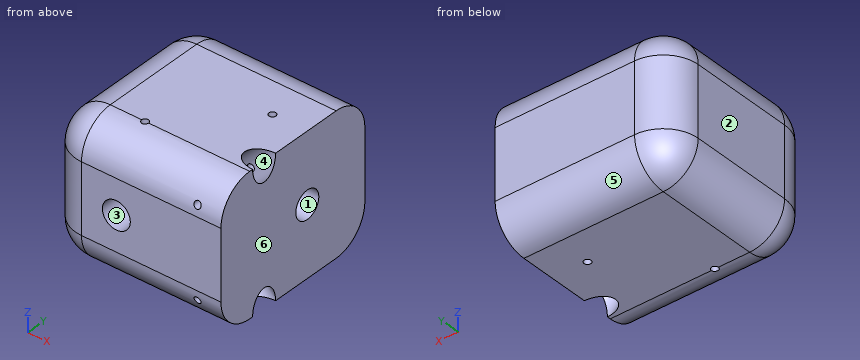
from build123d import *

# Parameters (mm, degrees)
F0_W          = 30
F0_H          = 30
F1_DEPTH      = 20
F2_R          = 2
F3_DEPTH      = 15
F4_R          = 2
F4_R_2        = 0.5
F5_DEPTH      = 15
F7_R          = 2
F8_DEPTH      = 15
F10_R         = 2
F11_DEPTH     = 15
F12_R         = 0.5
F13_DEPTH     = 20.0010001
F14_T1_DEPTH  = 10
F14_T3_DEPTH  = 32.5
F14_T5_DEPTH  = 15
F14_S9_W      = 5
F14_S9_H      = 5
F14_T10_DEPTH = 5
F14_S15_W     = 5
F14_S15_H     = 5
F14_T16_DEPTH = 5
F14_S21_W     = 5
F14_S21_H     = 5
F14_T22_DEPTH = 5
F14_S27_W     = 5
F14_S27_H     = 5
F14_T28_DEPTH = 5


# Not quite as in the source:
# - a fillet or chamfer that OpenCascade refuses, or shapes differently, is made with other operations: its cross-section is extruded or revolved along the edge and cut away or added


with BuildPart() as f1:
    # F0 (on Top) → F1 (new body)
    with BuildSketch(Plane.XY):
        Rectangle(F0_W, F0_H)
    extrude(amount=F1_DEPTH)

    # F2 (on face) → F3 (cut)
    with BuildSketch(Plane.YZ.offset(15)):
        with Locations((0, 10)):
            Circle(F2_R)
    extrude(amount=-F3_DEPTH, mode=Mode.SUBTRACT)

    # F4 (on face) → F5 (cut)
    with BuildSketch(Plane.XZ.offset(15)):
        with Locations((0, 10)):
            Circle(F4_R)
        with Locations((11.4644660941, 16.4644660941)):
            Circle(F4_R_2)
        with Locations((11.4644660941, 3.5355339059)):
            Circle(F4_R_2)
    extrude(amount=-F5_DEPTH, mode=Mode.SUBTRACT)

    # F7 (on face) → F8 (cut)
    with BuildSketch(Plane(origin=(17.5, 0, 17.5), x_dir=(0, 1, 0), z_dir=(0.7071067812, 0, 0.7071067812))):
        with Locations((-7.5, 3.5355339059)):
            Circle(F7_R)
    extrude(amount=-F8_DEPTH, mode=Mode.SUBTRACT)

    # F10 (on face) → F11 (cut)
    with BuildSketch(Plane(origin=(7.5, 0, -7.5), x_dir=(0.7071067812, 0, 0.7071067812), z_dir=(0.7071067812, 0, -0.7071067812))):
        with Locations((10.6066017178, 7.5)):
            Circle(F10_R)
    extrude(amount=-F11_DEPTH, mode=Mode.SUBTRACT)

    # F12 (on face) → F13 (cut, through all)
    with BuildSketch(Plane.XY.offset(20)):
        Polygon((-60, -15), (-10, -15), (-10, 10), (15, 10), (15, 50), (-60, 50), align=None)
        with Locations((10, 0)):
            Circle(F12_R)
        with Locations((0, -10)):
            Circle(F12_R)
    extrude(amount=-F13_DEPTH, mode=Mode.SUBTRACT)

    # F14: fillet of radius 5 on 8 edges, made by hand

    # F14_s2 → F14_t1 (cut)
    with BuildSketch(Plane.XY.offset(5)):
        with BuildLine():
            ThreePointArc((-5, -15), (-8.5355339059, -13.5355339059), (-10, -10))
            Line((-10, -10), (-10, -15))
            Line((-10, -15), (-5, -15))
        make_face()
        with BuildLine():
            ThreePointArc((-5, 10), (-8.5355339059, 8.5355339059), (-10, 5))
            Line((-10, 5), (-10, 10))
            Line((-10, 10), (-5, 10))
        make_face()
    extrude(amount=F14_T1_DEPTH, mode=Mode.SUBTRACT)

    # F14_s4 → F14_t3 (cut)
    with BuildSketch(Plane.YZ.offset(-5)):
        with BuildLine():
            ThreePointArc((-10, 20), (-13.5355339059, 18.5355339059), (-15, 15))
            Line((-15, 15), (-15, 20))
            Line((-15, 20), (-10, 20))
        make_face()
        with BuildLine():
            ThreePointArc((10, 15), (8.5355339059, 18.5355339059), (5, 20))
            Line((5, 20), (10, 20))
            Line((10, 20), (10, 15))
        make_face()
        with BuildLine():
            ThreePointArc((5, 0), (8.5355339059, 1.4644660941), (10, 5))
            Line((10, 5), (10, 0))
            Line((10, 0), (5, 0))
        make_face()
        with BuildLine():
            ThreePointArc((-10, 0), (-13.5355339059, 1.4644660941), (-15, 5))
            Line((-15, 5), (-15, 0))
            Line((-15, 0), (-10, 0))
        make_face()
    extrude(amount=F14_T3_DEPTH, mode=Mode.SUBTRACT)

    # F14_s6 → F14_t5 (cut)
    with BuildSketch(Plane.XZ.offset(-5)):
        with BuildLine():
            ThreePointArc((-5, 20), (-8.5355339059, 18.5355339059), (-10, 15))
            Line((-10, 15), (-10, 20))
            Line((-10, 20), (-5, 20))
        make_face()
        with BuildLine():
            ThreePointArc((-5, 0), (-8.5355339059, 1.4644660941), (-10, 5))
            Line((-10, 5), (-10, 0))
            Line((-10, 0), (-5, 0))
        make_face()
    extrude(amount=F14_T5_DEPTH, mode=Mode.SUBTRACT)


with BuildPart() as f14_tool8:
    # F14_s9 → F14_t10 (new body)
    with BuildSketch(Plane.YZ.offset(-5)):
        with Locations((-12.5, 17.5)):
            Rectangle(F14_S9_W, F14_S9_H)
    extrude(amount=-F14_T10_DEPTH)

    # F14_s11 → F14_t12 (revolve, cut)
    with BuildSketch(Plane(origin=(-5, -10, 15), x_dir=(0, 0.7071067812, -0.7071067812), z_dir=(0, 0.7071067812, 0.7071067812))):
        with BuildLine():
            ThreePointArc((0, -5), (5, 0), (0, 5))
            Line((0, 5), (0, -5))
        make_face()
    revolve(axis=Axis((-5, -10, 15), (-1, 0, 0)), mode=Mode.SUBTRACT)


with BuildPart() as f1_1:
    add(f1.part)

    # F14_t7: cut F14_tool8
    add(f14_tool8.part, mode=Mode.SUBTRACT)


with BuildPart() as f14_tool14:
    # F14_s15 → F14_t16 (new body)
    with BuildSketch(Plane.YZ.offset(-5)):
        with Locations((-12.5, 2.5)):
            Rectangle(F14_S15_W, F14_S15_H)
    extrude(amount=-F14_T16_DEPTH)

    # F14_s17 → F14_t18 (revolve, cut)
    with BuildSketch(Plane(origin=(-5, -10, 5), x_dir=(0, 0.7071067812, 0.7071067812), z_dir=(0, -0.7071067812, 0.7071067812))):
        with BuildLine():
            ThreePointArc((0, -5), (5, 0), (0, 5))
            Line((0, 5), (0, -5))
        make_face()
    revolve(axis=Axis((-5, -10, 5), (-1, 0, 0)), mode=Mode.SUBTRACT)


with BuildPart() as f1_2:
    add(f1_1.part)

    # F14_t13: cut F14_tool14
    add(f14_tool14.part, mode=Mode.SUBTRACT)


with BuildPart() as f14_tool20:
    # F14_s21 → F14_t22 (new body)
    with BuildSketch(Plane.YZ.offset(-5)):
        with Locations((7.5, 17.5)):
            Rectangle(F14_S21_W, F14_S21_H)
    extrude(amount=-F14_T22_DEPTH)

    # F14_s23 → F14_t24 (revolve, cut)
    with BuildSketch(Plane(origin=(-5, 5, 15), x_dir=(0, -0.7071067812, -0.7071067812), z_dir=(0, 0.7071067812, -0.7071067812))):
        with BuildLine():
            ThreePointArc((0, -5), (5, 0), (0, 5))
            Line((0, 5), (0, -5))
        make_face()
    revolve(axis=Axis((-5, 5, 15), (-1, 0, 0)), mode=Mode.SUBTRACT)


with BuildPart() as f1_3:
    add(f1_2.part)

    # F14_t19: cut F14_tool20
    add(f14_tool20.part, mode=Mode.SUBTRACT)


with BuildPart() as f14_tool26:
    # F14_s27 → F14_t28 (new body)
    with BuildSketch(Plane.YZ.offset(-5)):
        with Locations((7.5, 2.5)):
            Rectangle(F14_S27_W, F14_S27_H)
    extrude(amount=-F14_T28_DEPTH)

    # F14_s29 → F14_t30 (revolve, cut)
    with BuildSketch(Plane(origin=(-5, 5, 5), x_dir=(0, -0.7071067812, 0.7071067812), z_dir=(0, -0.7071067812, -0.7071067812))):
        with BuildLine():
            ThreePointArc((0, -5), (5, 0), (0, 5))
            Line((0, 5), (0, -5))
        make_face()
    revolve(axis=Axis((-5, 5, 5), (-1, 0, 0)), mode=Mode.SUBTRACT)


with BuildPart() as f1_4:
    add(f1_3.part)

    # F14_t25: cut F14_tool26
    add(f14_tool26.part, mode=Mode.SUBTRACT)


solid = f1_4.part
The listing builds one solid part. Answer for the finished solid, in the listing's coordinates (mm). Face numbers are marked on the shaded views. A direction names the side the tool comes from. Round coordinates to 2 decimals unless told otherwise and drop trailing zeros. Order: outer loops, then holes, each group sorted by start corner. A loop starts at its lowest first (then second) coordinate and runs counter-clockwise, first axis right, second up. Notation, with made-up numbers: (46, 16) - (99, 16) arc R28 ccw to (99, 38) - close; hole circle Ø9 at (3, 6). An arc over 180 degrees is marked (long way). Write item = value, one per line. Start each with the question number.
1) For the marked faces 1, 2 and 3, determine the directions among +Z, -Z, +X, -X, +Y, -Y from which every point of the face is accessible in a straight line to the end or side of a thin tool.
2) Section C-C, the plane y = 3.25 is taken. Write down the section's boundary in (x, z), plus the area to 3 significant figures.
3) Given pin 1 (4.5 mm diameter, centred on y = 0, z = 10, fed in from +X); pin 2 (0.5 mm diameter, centred on x = 11.5, z = 16.5, fed in from -Y); pin 3 (0.6 mm diameter, centred on y = 1, z = 9, fed in from +X); pin 4 (1.1 mm diameter, centred on x = 11.5, z = 3.5, fed in from -Y), each flat-ended and moving along its own axis, determine where each tip first touches the part or whether it passes through.
4) Section A-A, the plane y = -5 is taken. Write down the section's boundary in (x, z), plus the area to 3 significant figures.
5) Straight lines are drawn through the part: L1, parallel to Y at x = 9.75, z = 5.75; L2, parallel to Y at x = 6, z = 8.5; L3, parallel to Z at x = 0, y = -5.5. For each, find the intervals that lie inside material, in ascending order.
6) Section B-B, the plane x = 10 is taken. Count the separate pieces of the cut face and the enclosed holes in it, plus the area to 3 significant figures.
7) For a pull along X with two mould halves and no side action, classify the marked faces 4, 5 and 6 as released by +X, released by -X, zero draft, split by the parting line, or undercut.
Results list:
q1.face_1 = +X
q1.face_2 = +Z, -Z, -X, +Y, -Y
q1.face_3 = -Y
q2.outline = (-10, 5) arc R5 ccw to (-5, 0) - (15, 0) - (15, 20) - (-5, 20) arc R5 ccw to (-10, 15) - close
q2.area = 489 mm^2
q3.pin_1 = 15
q3.pin_2 = 0
q3.pin_3 = 0
q3.pin_4 = -14.91
q4.outline = (-10, 5) arc R5 ccw to (-5, 0) - (15, 0) - (15, 20) - (-5, 20) arc R5 ccw to (-10, 15) - close; hole circle Ø4 at (0, 10); hole circle Ø1 at (11.46, 3.54); hole circle Ø1 at (11.46, 16.46)
q4.area = 475 mm^2
q5.L1 = -15 to -9.47, -5.53 to -0.43, 0.43 to 10
q5.L2 = -15 to -9.47, -5.53 to -1.32, 1.32 to 10
q5.L3 = 0 to 8, 12 to 20
q6.separate_pieces = 2
q6.enclosed_holes = 2
q6.area = 414 mm^2
q7.face_4 = undercut
q7.face_5 = zero draft
q7.face_6 = released by +X
